```python
from build123d import *

# Parameters (mm, degrees)
F0_R     = 3
F0_R_2   = 1.5
F1_DEPTH = 15
F2_DEPTH = 8
F3_SIZE  = 0.5
F4_W     = 1
F4_H     = 2
F5_DEPTH = 12.5


with BuildPart() as f1:
    # F0 (on Top) → F1 (new body)
    with BuildSketch(Plane.XY):
        Circle(F0_R)
        Circle(F0_R_2, mode=Mode.SUBTRACT)
    extrude(amount=F1_DEPTH)

    # F0 (on Top) → F2 (join)
    with BuildSketch(Plane.XY):
        Circle(F0_R_2)
    extrude(amount=F2_DEPTH)

    # F3
    f3_edges = [f1.edges().sort_by_distance(p)[0] for p in [
        (-3, 0, 0),
        (-3, 0, 15),
    ]]
    chamfer(f3_edges, length=F3_SIZE)

    # F4 (on Front) → F5 (cut, symmetric)
    with BuildSketch(Plane.XZ):
        Rectangle(F4_W, F4_H)
    extrude(amount=F5_DEPTH, both=True, mode=Mode.SUBTRACT)


solid = f1.part
```
The listing builds one solid part. Answer for the finished solid, in the listing's coordinates (mm). A direction names the side the tool comes from. Give positions to 0.01 mm unless a question says otherwise; leave off trailing zeros. Order: outer loops, then holes, each group sorted by start corner. A loop starts at its lowest first (then second) coordinate and runs counter-clockwise, first axis right, second up. Notation, with made-up numbers: (63, 12) - (97, 12) arc R21 cw to (97, 23) - close; hole circle Ø6 at (-38, 13). An arc over 180 degrees is marked (long way). Answer in a Markdown table with one row per item. Add a question column.
Q1. The part is cut by section B-B (y = 0). Determine the outline of the cut face in (x, z).
Q2. Find the intervals of material crossed by line 1 along Y through (x, z) = (0, 13.25); line 2 along Y through (x, z) = (0.6, 9.25); line 3 along X through (y, z) = (-2.6, 3.5), in increasing order. Write a range as [from, to].
Q3. The part is cut by section C-C (z = 11.25). Determine the outline of the cut face in (x, y).
Q4. The part is cut by section A-A (x = 0). Determine the outline of the cut face in (y, z), then the cut area to 4 significant figures.
Q5. Which of the six approach directions +Z, -Z, +X, -X, +Y, -Y give full straight-line access (tool end or side, diameter ignored) to faces 4 (the cylindrical face through (-1.5, 0.07, 11.45)), 5 (the flat face through (-0.5, 0, 0.5)), 6 (the conical face through (2.64, -0.05, 0.14))?
Q6. The part is cut by section D-D (z = 6.75). Determine the outline of the cut face in (x, y), then the cut area to 3 significant figures.
Q7. Given P1, Ø1.1, axis at y = 1, z = 0.5, coming from the -X side; P2, Ø0.8, axis at y = -1.5, z = 0.5, coming from the +X side, each flat-ended and moving along its own axis, determine where each tip first touches the part or whether it passes through.
Q8. For a pull along X with two mould halves and no side action, classify faces 1 (the flat face through (0.5, 0, 0.5)), 2 (the flat face through (-1, 0, 0)), 3 (the conical face through (-2.64, 0.05, 0.14)) as released by +X, released by -X, zero draft, split by the parting line, or undercut.
Determined:
| question | item | result |
|---|---|---|
| 1 | outline | (-3, 0.5) - (-2.5, 0) - (-0.5, 0) - (-0.5, 1) - (0.5, 1) - (0.5, 0) - (2.5, 0) - (3, 0.5) - (3, 14.5) - (2.5, 15) - (1.5, 15) - (1.5, 8) - (-1.5, 8) - (-1.5, 15) - (-2.5, 15) - (-3, 14.5) - close |
| 2 | line 1 | y = [-3, -1.5], [1.5, 3] |
| 2 | line 2 | y = [-2.94, -1.37], [1.37, 2.94] |
| 2 | line 3 | x = [-1.5, 1.5] |
| 3 | outline | circle Ø6 at (0, 0); hole circle Ø3 at (0, 0) |
| 4 | outline | (-3, 1) - (3, 1) - (3, 14.5) - (2.5, 15) - (1.5, 15) - (1.5, 8) - (-1.5, 8) - (-1.5, 15) - (-2.5, 15) - (-3, 14.5) - close |
| 4 | area | 62.75 mm² |
| 5 | face 4 | +Z |
| 5 | face 5 | -Z, +Y, -Y |
| 5 | face 6 | -Z, +X |
| 6 | outline | circle Ø6 at (0, 0) |
| 6 | area | 28.3 mm² |
| 7 | P1 | stops at x = -2.97 |
| 7 | P2 | stops at x = 2.79 |
| 8 | face 1 | undercut |
| 8 | face 2 | zero draft |
| 8 | face 3 | released by -X |
